Study the drawing (mm; zero at the part's minimum x, y, z) and answer. A direction names the side the tool comes from. Round coordinates to 2 decimals unless told otherwise and drop trailing zeros. Loops run counter-clockwise (first coordinate to the right, second up) from the corner with the lowest first, then second, coordinate; pieces in that order, holes last. Notation, with made-up numbers: M 47.25,1.5 L 53.25,1.5 A34 ccw 53.25,36.5 Z; hole C -7,-2.75 d1. An arc over 180 degrees is marked long. Write each question's results on one line, items separated by ' | '.
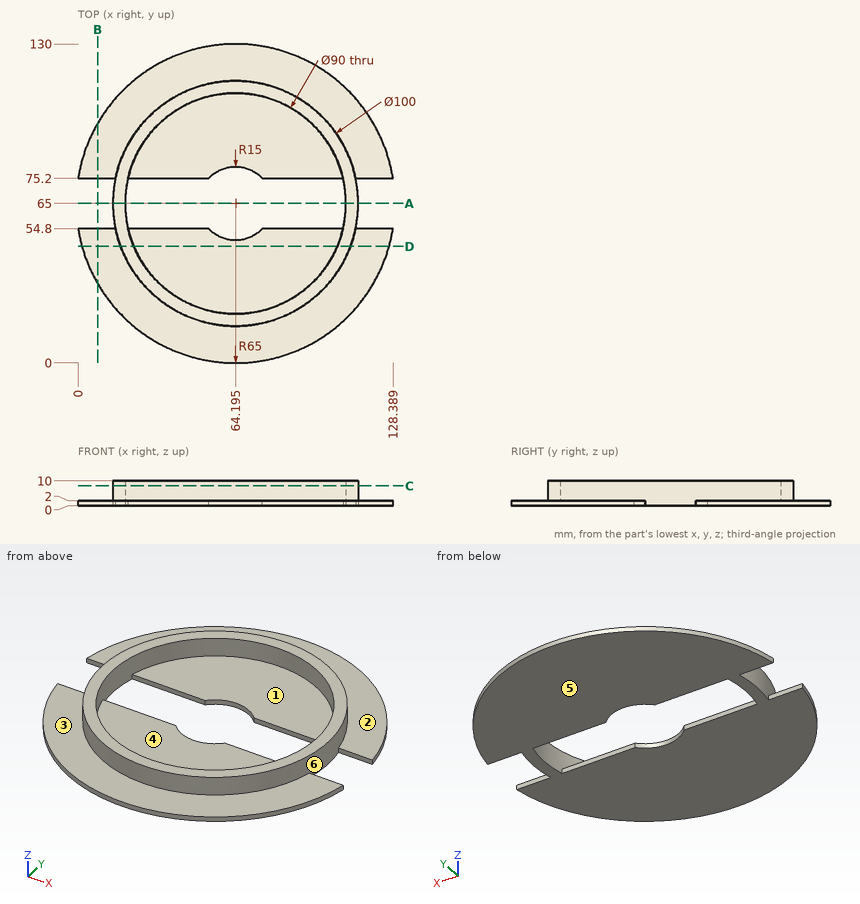
Item 1: Straight lines are drawn through the part: line 1 (X direction, y = 65, z = 2.25) (1 decimal); line 2 (Y direction, x = 30.5, z = 4.5) (1 decimal); line 3 (Z direction, x = 58, y = 91). For each, find the intervals that lie inside material, in ascending order.
Outcome:
line 1: x = 14.2 to 19.2, 109.2 to 114.2 | line 2: y = 28.1 to 35.2, 94.8 to 101.9 | line 3: z = 0 to 2
Item 2: The part is cut by section C-C (z = 8). Determine the outline of the cut face in (x, y) (1 decimal), plus the area to 3 significant figures.
Outcome:
outline: C 64.2,65 d100; hole C 64.2,65 d90 | area: 1,490 mm2
Item 3: The mould has two halves that part along X. Classify the marked faces 4, 5 and 6: pulls with the +X half, pulls with the -X half, needs draft (parallel to the pull), parting line crosses it, or undercut.
Outcome:
face 4: undercut | face 5: needs draft | face 6: parting line crosses it
Item 4: Flat-ended cylindrical pins translate along their axes: pin 1 (1 mm diameter, centred on x = 122, z = 1, fed in from -Y) (1 decimal); pin 2 (16.5 mm diameter, centred on x = 92.5, y = 95.5, fed in from +Z); pin 3 (1 mm diameter, centred on x = 11, z = 1, fed in from +Y) (1 decimal); pin 4 (1 mm diameter, centred on x = 87, z = 1, fed in from -Y). Find the tip coordinate at first contact, or state that the pin passes through.
Outcome:
pin 1: stops at y = 34.3 | pin 2: stops at z = 10 | pin 3: stops at y = 103.1 | pin 4: stops at y = 3.95
Item 5: The part is cut by section B-B (x = 8). Determine the outline of the cut face in (y, z).
Outcome:
outline: M 32.33,0 L 54.8,0 L 54.8,2 L 32.33,2 Z; M 75.2,0 L 97.67,0 L 97.67,2 L 75.2,2 Z
Item 6: The part is cut by section A-A (y = 65). Determine the outline of the cut face in (x, z) (1 decimal), plus the area to 3 significant figures.
Outcome:
outline: M 14.2,0 L 19.2,0 L 19.2,10 L 14.2,10 Z; M 109.2,0 L 114.2,0 L 114.2,10 L 109.2,10 Z | area: 100 mm2
Item 7: The part is cut by section D-D (y = 47.5). Determine the outline of the cut face in (x, z) (1 decimal).
Outcome:
outline: M 1.6,0 L 126.8,0 L 126.8,2 L 111,2 L 111,10 L 105.7,10 L 105.7,2 L 22.7,2 L 22.7,10 L 17.4,10 L 17.4,2 L 1.6,2 Z
Item 8: For the marked faces 1, 2 and 3, determine the directions among +Z, -Z, +X, -X, +Y, -Y from which every point of the face is accessible in a straight line to the end or side of a thin tool.
Outcome:
face 1: +Z | face 2: +Z, +Y | face 3: +Z, -Y
